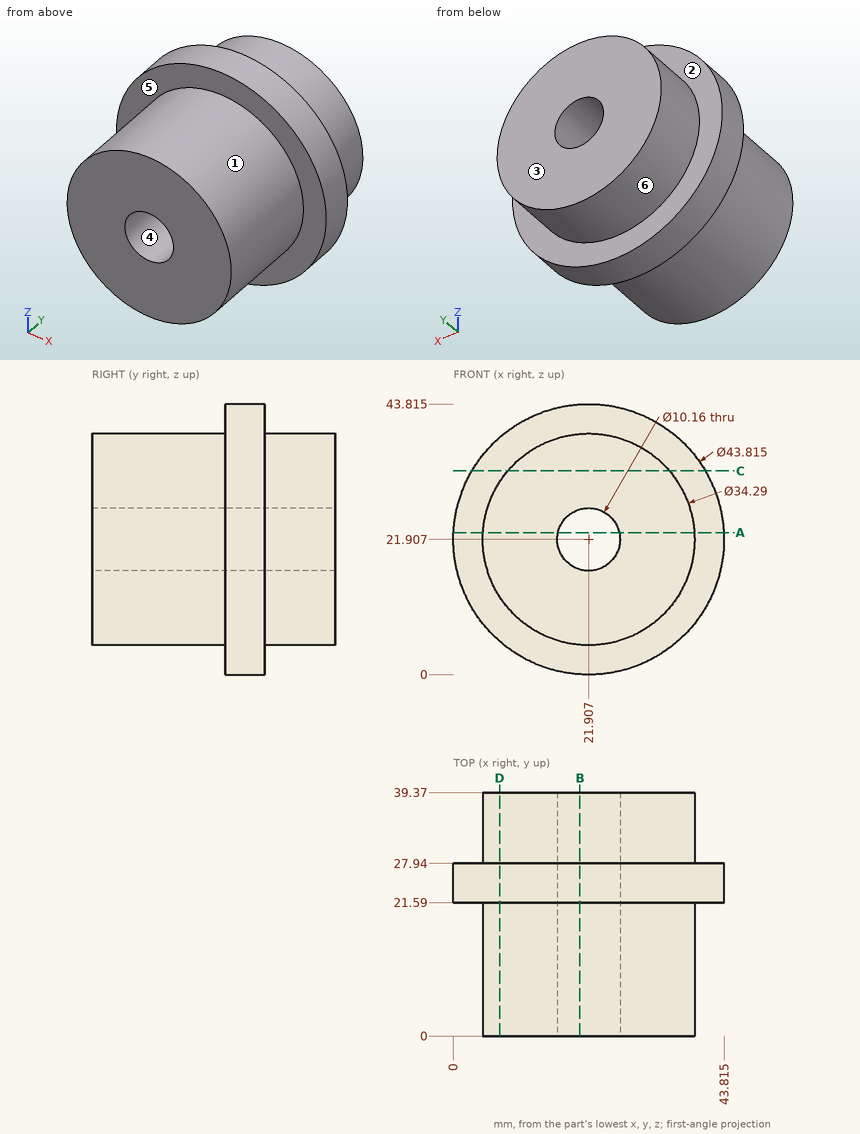
The drawing under review shows one solid part. Ordinate dimensions are in mm from its lowest x, y, z. A direction names the side the tool comes from. Give positions to 0.01 mm unless a question says otherwise; leave off trailing zeros. Loops run counter-clockwise (first coordinate to the right, second up) from the corner with the lowest first, then second, coordinate; pieces in that order, holes last. Notation, with made-up numbers: M -22.5,41.5 L -8.5,41.5 A17 cw -8.5,46.5 Z; hole C 28.5,-8 d3. An arc over 180 degrees is marked long. Return JSON: item names as keys, results as strings. Group by question number.
Item 1: We need section C-C (z = 33). Give the boundary of the cut face in (x, y) (1 decimal), and give its area (3 significant figures).
Item 2: Mouldability with a two-part tool opening along X and no side actions: class the marked faces 4, 5 and 6 as released by +X, released by -X, zero draft, split by the parting line, or undercut.
Item 3: We need section D-D (x = 7.5). Give the boundary of the cut face in (y, z) (1 decimal).
Item 4: We need section A-A (z = 23). Give the boundary of the cut face in (x, y).
Item 5: Tool access review of the marked faces 1, 2 and 3: name each direction out of +Z, -Z, +X, -X, +Y, -Y from which nothing blocks a thin tool from reaching the whole face with its end or side.
Item 6: For probe 1 along Y at (x, z) = (28, 4.5); probe 2 along Z at (x, y) = (34, 7.5) (1 decimal); probe 3 along Z at (x, y) = (21, 32) (1 decimal), list the stretches that pass through material, from the lowest coordinate up.
Item 7: We need section B-B (x = 20.5). Give the boundary of the cut face in (y, z) (1 decimal).
Item 8: Insertion check: pin 1 Ø3 at (y, z) = (14, 19) entering from +X (1 decimal); pin 2 Ø8 at (y, z) = (34, 32) entering from +X; pin 3 Ø3 at (y, z) = (30, 17) entering from +X. Each pin has a flat end and moves straight along its axis. Give the tip position at first contact, or say it passes through.
Output:
{
 "1": {"outline": "M 3,21.6 L 8.8,21.6 L 8.8,0 L 35,0 L 35,21.6 L 40.8,21.6 L 40.8,27.9 L 35,27.9 L 35,39.4 L 8.8,39.4 L 8.8,27.9 L 3,27.9 Z", "area": "1,100 mm^2"},
 "2": {"face 4": "undercut", "face 5": "zero draft", "face 6": "split by the parting line"},
 "3": {"outline": "M 0,12.6 L 21.6,12.6 L 21.6,5.4 L 27.9,5.4 L 27.9,12.6 L 39.4,12.6 L 39.4,31.2 L 27.9,31.2 L 27.9,38.4 L 21.6,38.4 L 21.6,31.2 L 0,31.2 Z"},
 "4": {"outline": "M 0.03,21.59 L 4.8,21.59 L 4.8,0 L 16.95,0 L 16.95,39.37 L 4.8,39.37 L 4.8,27.94 L 0.03,27.94 Z; M 26.87,0 L 39.02,0 L 39.02,21.59 L 43.79,21.59 L 43.79,27.94 L 39.02,27.94 L 39.02,39.37 L 26.87,39.37 Z"},
 "5": {"face 1": "-Y", "face 2": "+Y", "face 3": "+Z, -Z, +X, -X, +Y"},
 "6": {"probe 1": "y = 21.59 to 27.94", "probe 2": "z = 9.8 to 34.1", "probe 3": "z = 4.8 to 16.9, 26.9 to 39"},
 "7": {"outline": "M 0,4.8 L 21.6,4.8 L 21.6,0 L 27.9,0 L 27.9,4.8 L 39.4,4.8 L 39.4,17 L 0,17 Z; M 0,26.8 L 39.4,26.8 L 39.4,39 L 27.9,39 L 27.9,43.8 L 21.6,43.8 L 21.6,39 L 0,39 Z"},
 "8": {"pin 1": "stops at x = 39", "pin 2": "stops at x = 37.93", "pin 3": "stops at x = 38.71"}
}
